from build123d import *

# Parameters (mm, degrees)
F0_W     = 1397
F0_H     = 889
F1_DEPTH = 1270
F2_W     = 635
F2_H     = 635
F3_DEPTH = 1397.001
F4_W     = 762
F4_H     = 508
F5_DEPTH = 635.001
F6_W     = 762
F6_H     = 127
F7_DEPTH = 127


with BuildPart() as f1:
    # F0 (on Front) → F1 (new body)
    with BuildSketch(Plane.XZ):
        Rectangle(F0_W, F0_H)
    extrude(amount=F1_DEPTH)

    # F2 (on face) → F3 (cut, through all)
    with BuildSketch(Plane.YZ.offset(698.5)):
        with Locations((-952.5, 127)):
            Rectangle(F2_W, F2_H)
    extrude(amount=-F3_DEPTH, mode=Mode.SUBTRACT)

    # F4 (on face) → F5 (cut, through all)
    with BuildSketch(Plane.XZ.offset(635)):
        with Locations((317.5, 190.5)):
            Rectangle(F4_W, F4_H)
    extrude(amount=-F5_DEPTH, mode=Mode.SUBTRACT)

    # F6 (on face) → F7 (cut)
    with BuildSketch(Plane.XZ.offset(635)):
        with Locations((317.5, -127)):
            Rectangle(F6_W, F6_H)
    extrude(amount=-F7_DEPTH, mode=Mode.SUBTRACT)


solid = f1.part
Work out the finished part from the listing and answer in its coordinate system (mm). A direction names the side the tool comes from. Give positions to 0.01 mm unless a question says otherwise; leave off trailing zeros. Write each loop counter-clockwise with the first axis right and the second up, starting at its lowest first coordinate (ties: lowest second). Pieces come first, ordered by that corner, then holes. Notation, with made-up numbers: (-4, 54.5) - (14, 54.5) arc R18 cw to (14, 59.5) - close; hole circle Ø1 at (40.25, 35.25). An arc over 180 degrees is marked (long way). One line per item, written item: value. Start each with the question number.
1. Find section C-C (z = 26). Write down the section's boundary in (x, y), then the cut area to 3 significant figures.
2. For faces 1 (the flat face through (-10, -1270, -316)), 2 (the flat face through (698.5, -626, -299)), 3 (the flat face through (-377, -635, 123)), 4 (the flat face through (312, -258, -63.5)), 5 (the flat face through (312, -508, -126)), determine the directions among +Z, -Z, +X, -X, +Y, -Y from which every point of the face is accessible in a straight line to the end or side of a thin tool.
3. Find section D-D (y = -791). Write down the section's boundary in (x, z), then the cut area to 3 significant figures.
4. Given pin 1 (4 mm diameter, centred on x = 233.5, z = -148.5, fed in from -Y); pin 2 (6 mm diameter, centred on y = -446.5, z = 203, fed in from +X); pin 3 (8 mm diameter, centred on x = -377.5, z = -54, fed in from -Y), each flat-ended and moving along its own axis, determine where each tip first touches the part or whether it passes through.
5. Find section A-A (y = -567.5). Write down the section's boundary in (x, z).
6. Find section B-B (x = 121.5). Write down the section's boundary in (y, z), then the cut area to 3 significant figures.
7. Consider probe 1 along Z at (x, y) = (-567.5, -1132); probe 2 along X at (y, z) = (-148.5, 151); probe 3 along Z at (x, y) = (281.5, -448). Determine where each line is inside the solid, lowest interval first.
Geometry results:
1. outline: (-698.5, -635) - (-63.5, -635) - (-63.5, 0) - (-698.5, 0) - close
1. area: 403,000 mm2
2. face 1: +Z, -Z, +X, -X, -Y
2. face 2: +Z, -Z, +X, +Y, -Y
2. face 3: +Z, +X, -X, -Y
2. face 4: +Z, +X, +Y, -Y
2. face 5: +Z, +X, -Y
3. outline: (-698.5, -444.5) - (698.5, -444.5) - (698.5, -190.5) - (-698.5, -190.5) - close
3. area: 355,000 mm2
4. pin 1: y = -508
4. pin 2: x = -63.5
4. pin 3: y = -635
5. outline: (-698.5, -444.5) - (698.5, -444.5) - (698.5, -190.5) - (-63.5, -190.5) - (-63.5, 444.5) - (-698.5, 444.5) - close
6. outline: (-1270, -444.5) - (0, -444.5) - (0, -63.5) - (-508, -63.5) - (-508, -190.5) - (-1270, -190.5) - close
6. area: 387,000 mm2
7. probe 1: -444.5 to -190.5
7. probe 2: -698.5 to -63.5
7. probe 3: -444.5 to -63.5
